Design review of the part built by this model. Coordinates are the model's own, in mm. Face numbers are marked on the shaded views. A direction names the side the tool comes from. Give positions to 0.01 mm unless a question says otherwise; leave off trailing zeros. Write each loop counter-clockwise with the first axis right and the second up, starting at its lowest first coordinate (ties: lowest second). Pieces come first, ordered by that corner, then holes. Notation, with made-up numbers: (14.5, 83) -> (39.5, 83) arc R12 cw to (39.5, 93) -> close; hole circle Ø9 at (11, 50). An arc over 180 degrees is marked (long way). Write each question's results on one line, items separated by ' | '. Start each with the question number.
(1) Mouldability with a two-part tool opening along Y and no side actions: class the marked faces 1, 2, 3 and 4 as released by +Y, released by -Y, zero draft, split by the parting line, or undercut.
(2) To check wall thickness, follow probe 1 along Y at (x, z) = (0, 2); probe 2 along Y at (x, z) = (0, 12.3); probe 3 along Z at (x, y) = (0.5, 2.25). State the ranges of each line that lie inside material, in increasing order.
(3) Take a section at A-A (y = 0). State the section outline as (x, z) points.
(4) Take a section at C-C (z = 9). State the section outline as (x, y) points.
(5) Clearance check with flat-ended pins moving along their axes: pin 1 (3.5 mm diameter, centred on x = 0, y = 0, fed in from +Z); pin 2 (5 mm diameter, centred on x = -2, z = 9, fed in from +Y). State where each tip first meets the part, or that it passes through.
(6) For the marked faces 5 and 6, list the 3-axis set-ups (+Z, -Z, +X, -X, +Y, -Y) from which the entire face can be reached by the end or side of a thin tool; tool diameter is ignored.
(7) Take a section at D-D (y = -3.5). State the section outline as (x, z) points, plus the area to 3 significant figures.
from build123d import *

# Parameters (mm, degrees)
F0_R     = 4
F1_DEPTH = 11
F2_R     = 5.5
F2_R_2   = 4
F3_DEPTH = 2
F4_R     = 2.85
F5_DEPTH = 3.5
F6_R     = 1.6
F7_DEPTH = 25


with BuildPart() as f1:
    # F0 (on Top) → F1 (new body)
    with BuildSketch(Plane.XY):
        Circle(F0_R)
    extrude(amount=F1_DEPTH)

    # F2 (on face) → F3 (join)
    with BuildSketch(Plane.XY.offset(11)):
        Circle(F2_R)
        Circle(F2_R_2, mode=Mode.SUBTRACT)
        Circle(F2_R_2)
    extrude(amount=F3_DEPTH)

    # F4 (on face) → F5 (cut)
    with BuildSketch(Plane.XY.offset(13)):
        Circle(F4_R)
    extrude(amount=-F5_DEPTH, mode=Mode.SUBTRACT)

    # F6 (on face) → F7 (cut)
    with BuildSketch(Plane.XY.offset(9.5)):
        Circle(F6_R)
    extrude(amount=-F7_DEPTH, mode=Mode.SUBTRACT)


solid = f1.part
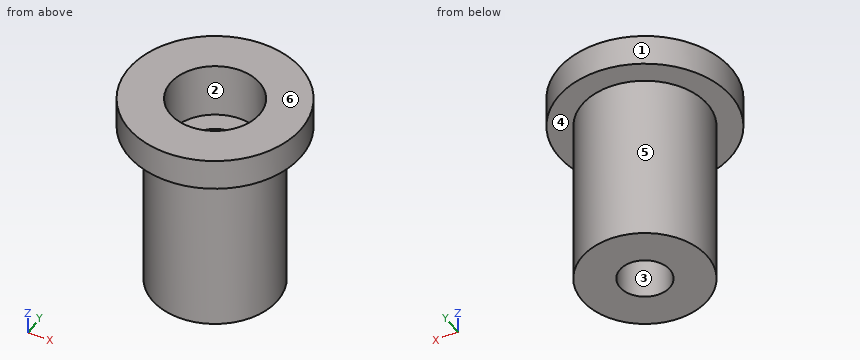
Report:
1) face 1: split by the parting line | face 2: undercut | face 3: undercut | face 4: zero draft
2) probe 1: -4 to -1.6, 1.6 to 4 | probe 2: -5.5 to -2.85, 2.85 to 5.5 | probe 3: 0 to 9.5
3) outline: (-5.5, 11) -> (-4, 11) -> (-4, 0) -> (-1.6, 0) -> (-1.6, 9.5) -> (-2.85, 9.5) -> (-2.85, 13) -> (-5.5, 13) -> close; (1.6, 0) -> (4, 0) -> (4, 11) -> (5.5, 11) -> (5.5, 13) -> (2.85, 13) -> (2.85, 9.5) -> (1.6, 9.5) -> close
4) outline: circle Ø8 at (0, 0); hole circle Ø3.2 at (0, 0)
5) pin 1: z = 9.5 | pin 2: y = 5.48
6) face 5: -Z | face 6: +Z, +X, -X, +Y, -Y
7) outline: (-4.24, 11) -> (-1.94, 11) -> (-1.94, 0) -> (1.94, 0) -> (1.94, 11) -> (4.24, 11) -> (4.24, 13) -> (-4.24, 13) -> close | area: 59.6 mm2
